Check sheet for the modelled part. Datum: model origin and axes. Units: mm. A direction names the side the tool comes from. Round coordinates to 2 decimals unless told otherwise and drop trailing zeros.
Item 1: Section check A-A, the plane z = 0.5. State how many separate pieces and enclosed holes the cut face has, plus the area to 3 significant figures.
Item 2: Material ranges on line 1 along X through (y, z) = (-0.75, -4); line 2 along X through (y, z) = (-0.25, -6); line 3 along X through (y, z) = (-2, 5.5), recorded low to high.
Item 3: Set-up check for faces 4 (the flat face through (1.57, -5.55, -3.43)), 5 (the flat face through (-9.5, -0.5, -0.1)): record each of +Z, -Z, +X, -X, +Y, -Y from which the full face is reachable in a straight line by a thin tool's end or side.
Item 4: Release check for a two-part mould opening along Y. For faces 1 (the flat face through (-19, -0.5, -0.1)), 2 (the flat face through (-9.821, -0.493, 5.596)), 3 (the flat face through (16.946, -0.493, 5.596)) record: pulls with the +Y half, pulls with the -Y half, needs draft (parallel to the pull), parting line crosses it, or undercut.
Item 5: Depth check by flat-ended pin: pin 1 (3 mm diameter, centred on y = -4.5, z = 0.5, fed in from -X) (3 decimals); pin 2 (1.5 mm diameter, centred on y = -4.5, z = 0.5, fed in from +X); pin 3 (3.5 mm diameter, centred on y = -3.5, z = -4.5, fed in from -X); pin 4 (0.8 mm diameter, centred on x = -17, y = -0.5, fed in from +Z). Enter the tip coordinate at first touch or a pass-through.
from build123d import *

# Parameters (mm, degrees)
F1_DEPTH      = 20
F1_DEPTH_BACK = 20
F3_DEPTH      = 24
F3_DEPTH_BACK = 24
F4_W          = 0.375
F4_H          = 7.5
F5_DEPTH      = 0.5
F16_W         = 8.5
F16_H         = 10
F17_DEPTH     = 1
F18_DEPTH     = 1
F19_DEPTH     = 1


with BuildPart() as f1:
    # F0 (on Right) → F1 (new body, two sides)
    with BuildSketch(Plane.YZ) as f1_sk:
        Polygon((0, -7), (0, 0), (-6, 0), (-6, -3.75), align=None)
        Polygon((-6, 0), (0, 0), (0, 7), (-6, 3.75), align=None)
    extrude(amount=F1_DEPTH)
    extrude(f1_sk.sketch, amount=-F1_DEPTH_BACK)

    # F2 (on Right) → F3 (cut, two sides)
    with BuildSketch(Plane.YZ) as f3_sk:
        Polygon((-1, 5.8904322458), (-2.7620611939, 4.9370331568), (-6, 3.185080433), (-6, -3.185), (-1, -5.89), (-1, 0), align=None)
    extrude(amount=-F3_DEPTH, mode=Mode.SUBTRACT)
    extrude(f3_sk.sketch, amount=F3_DEPTH_BACK, mode=Mode.SUBTRACT)

    # F4 (on face) → F5 (join)
    with BuildSketch(Plane.XZ.offset(6)):
        with Locations((-0.1875, 0)):
            Rectangle(F4_W, F4_H)
        with Locations((0.1875, 0)):
            Rectangle(F4_W, F4_H)
        with Locations((6.6875, 0)):
            Rectangle(F4_W, F4_H)
        with Locations((6.3125, 0)):
            Rectangle(F4_W, F4_H)
        with Locations((13.1875, 0)):
            Rectangle(F4_W, F4_H)
        with Locations((12.8125, 0)):
            Rectangle(F4_W, F4_H)
        with Locations((19.6875, 0)):
            Rectangle(F4_W, F4_H)
        with Locations((19.3125, 0)):
            Rectangle(F4_W, F4_H)
        with Locations((-6.6875, 0)):
            Rectangle(F4_W, F4_H)
        with Locations((-6.3125, 0)):
            Rectangle(F4_W, F4_H)
        with Locations((-13.1875, 0)):
            Rectangle(F4_W, F4_H)
        with Locations((-12.8125, 0)):
            Rectangle(F4_W, F4_H)
        with Locations((-19.6875, 0)):
            Rectangle(F4_W, F4_H)
        with Locations((-19.3125, 0)):
            Rectangle(F4_W, F4_H)
    extrude(amount=-F5_DEPTH)

    # F7 (on offset) → F8 (revolve)
    with BuildSketch(Plane.XZ.offset(5.75)):
        Polygon((-13.086971221, -3.3170442338), (-19.1837764068, 3.4343508854), (-19.2789044945, 3.353184308), (-13.3750620526, -3.1845304184), (-13.1797424519, -3.4008207144), align=None)
    revolve(axis=Axis((-16.3269832736, -5.75, 0.0843269448), (-0.6702118448, 0, 0.7421698479)))

    # F7 (on offset) → F9 (revolve)
    with BuildSketch(Plane.XZ.offset(5.75)):
        Polygon((-6.586971221, -3.3170442338), (-12.6837764068, 3.4343508854), (-12.8043608498, 3.3254578575), (-12.7513883635, 3.2667979242), (-6.8750620526, -3.1845304184), (-6.6797424519, -3.4008207144), align=None)
    revolve(axis=Axis((-12.7778746067, -5.75, 3.2961278908), (-0.6702118448, 0, 0.7421698479)))

    # F7 (on offset) → F10 (revolve)
    with BuildSketch(Plane.XZ.offset(5.75)):
        Polygon((-6.2765476378, 3.3505744048), (-0.3750620526, -3.1845304184), (-0.1797424519, -3.4008207144), (-0.086971221, -3.3170442338), (-6.1837764068, 3.4343508854), align=None)
    revolve(axis=Axis((-3.3258048452, -5.75, 0.0830219932), (-0.6702118448, 0, 0.7421698479)))

    # F7 (on offset) → F11 (revolve)
    with BuildSketch(Plane.XZ.offset(5.75)):
        Polygon((0.086971221, -3.3170442338), (0.1797424519, -3.4008207144), (0.3750620526, -3.1845304184), (6.2765476378, 3.3505744048), (6.1837764068, 3.4343508854), align=None)
    revolve(axis=Axis((3.3258048452, -5.75, 0.0830219932), (0.6702118448, 0, 0.7421698479)))

    # F7 (on offset) → F12 (revolve)
    with BuildSketch(Plane.XZ.offset(5.75)):
        Polygon((12.7765476378, 3.3505744048), (12.6837764068, 3.4343508854), (6.586971221, -3.3170442338), (6.6797424519, -3.4008207144), (6.8750620526, -3.1845304184), align=None)
    revolve(axis=Axis((9.8258048452, -5.75, 0.0830219932), (0.6702118448, 0, 0.7421698479)))

    # F7 (on offset) → F13 (revolve)
    with BuildSketch(Plane.XZ.offset(5.75)):
        Polygon((19.2765476378, 3.3505744048), (19.1837764068, 3.4343508854), (13.086971221, -3.3170442338), (13.1797424519, -3.4008207144), (13.3750620526, -3.1845304184), align=None)
    revolve(axis=Axis((16.3258048452, -5.75, 0.0830219932), (0.6702118448, 0, 0.7421698479)))

    # F16 (on face) → F17 (cut)
    with BuildSketch(Plane(origin=(0, 0, 0), x_dir=(-1, 0, 0), z_dir=(0, 1, 0))):
        with Locations((-14.75, 0)):
            Rectangle(F16_W, F16_H)
        Polygon((-1, -5), (-1, 0), (-1, 5), (-9.5, 5), (-9.5, -5), align=None)
        Polygon((9.5, -5), (9.5, 5), (1, 5), (1, 0), (1, -5), align=None)
        with Locations((14.75, 0)):
            Rectangle(F16_W, F16_H)
    extrude(amount=-F17_DEPTH, mode=Mode.SUBTRACT)

    # F14 (on face) → F18 (cut)
    with BuildSketch(Plane(origin=(0, -2.9315436242, 5.4120805369), x_dir=(1, 0, 0), z_dir=(0, -0.4762831485, 0.8792919665))):
        Polygon((-15.5, 2.8339820398), (-19.5, 2.8339820398), (-19.5, -2.9896899922), (-10.375, -2.9896899922), align=None)
        Polygon((-10, -2.6014451901), (-4.75, 2.8339820398), (-14.75, 2.8339820398), align=None)
        Polygon((0, -2.9896899922), (0, 2.8339820398), (-4, 2.8339820398), (-9.625, -2.9896899922), align=None)
        Polygon((4, 2.8339820398), (0, 2.8339820398), (0, -2.9896899922), (9.625, -2.9896899922), align=None)
        Polygon((14.75, 2.8339820398), (4.75, 2.8339820398), (10, -2.6014451901), align=None)
        Polygon((19.5, -2.9896899922), (19.5, 2.8339820398), (15.5, 2.8339820398), (10.375, -2.9896899922), align=None)
    extrude(amount=-F18_DEPTH, mode=Mode.SUBTRACT)

    # F15 (on face) → F19 (cut)
    with BuildSketch(Plane(origin=(0, -2.9315436242, -5.4120805369), x_dir=(1, 0, 0), z_dir=(0, -0.4762831485, -0.8792919665))):
        Polygon((-19.501139431, 3.0074388159), (-19.501139431, -2.8162332161), (-10.376139431, -2.8162332161), (-15.501139431, 3.0074388159), align=None)
        Polygon((-10.001139431, -2.4279884139), (-4.751139431, 3.0074388159), (-14.751139431, 3.0074388159), align=None)
        Polygon((-0.001139431, -2.8162332161), (-0.001139431, 3.0074388159), (-4.001139431, 3.0074388159), (-9.626139431, -2.8162332161), align=None)
        Polygon((3.998860569, 3.0074388159), (-0.001139431, 3.0074388159), (-0.001139431, -2.8162332161), (0.4340025901, -2.8162332161), (9.623860569, -2.8162332161), align=None)
        Polygon((14.748860569, 3.0074388159), (4.748860569, 3.0074388159), (9.998860569, -2.4279884139), align=None)
        Polygon((19.498860569, -2.8162332161), (19.498860569, 3.0074388159), (15.498860569, 3.0074388159), (10.373860569, -2.8162332161), align=None)
    extrude(amount=-F19_DEPTH, mode=Mode.SUBTRACT)


solid = f1.part
Values found:
1. separate pieces: 18
1. enclosed holes: 1
1. area: 9.07 mm2
2. line 1: x = -20 to -19, -10.5 to -9.5, -1 to 1, 9.5 to 10.5, 19 to 20
2. line 2: x = -20 to -19.5, -10.53 to -9.45, 9.45 to 10.53, 19.5 to 20
2. line 3: x = -20 to -19.5, -13.76 to -13.03, -6.66 to -5.91, 5.91 to 6.66, 13.03 to 13.76, 19.5 to 20
3. face 4: none
3. face 5: +Y
4. face 1: needs draft
4. face 2: undercut
4. face 3: pulls with the -Y half
5. pin 1: stops at x = -19.875
5. pin 2: passes through
5. pin 3: stops at x = -20
5. pin 4: stops at z = 6.95
